Autodesk Inventor part; units mm, degrees
ref_plane "YZ Plane" through (0, 0, 0) normal (1, 0, 0) x (0, 1, 0)
ref_plane "XZ Plane" through (0, 0, 0) normal (0, 1, 0) x (-1, 0, 0)
ref_plane "XY Plane" through (0, 0, 0) normal (0, 0, 1) x (1, 0, 0)
sketch "Esboço1" plane through (0, 0, 0) normal (0, 0, 1) x (1, 0, 0)
  line L0 (-15, 15) -> (15, 15) construction
  line L1 (-15, 15) -> (-15, 10.6) construction
  line L2 (-15, 10.6) -> (-13, 10.6) construction
  line L3 (-13, 13.6) -> (-13, 10.6) construction
  line L4 (-13, 13.6) -> (-9.4247, 10.6) construction
  line L5 (-9.4247, 10.6) -> (-9.4247, 4.4) construction
  line L6 (-9.4247, 4.4) -> (-13, 1.4) construction
  line L7 (-13, 4.4) -> (-13, 1.4) construction
  line L8 (-15, 4.4) -> (-13, 4.4) construction
  line L9 (-15, 4.4) -> (-15, 0) construction
  line L10 (-15, 0) -> (0, 0) construction
  line L11 (-15, 4.4) -> (-14.5, 4.4) construction
  line L12 (-14.5, 4.4) -> (-14.5, 3.9)
  line L13 (-14.5, 3.9) -> (-15, 3.9)
  line L14 (-15, 3.9) -> (-15, 4.4) construction
  line L15 (-15, 10.6) -> (-14.5, 10.6) construction
  line L16 (-14.5, 10.6) -> (-14.5, 11.1)
  line L17 (-14.5, 11.1) -> (-15, 11.1)
  line L18 (-15, 11.1) -> (-15, 10.6) construction
  line L19 (-3.1, 9.4247) -> (3.1, 9.4247) construction
  line L20 (-6.1, 13) -> (-3.1, 9.4247) construction
  line L21 (-6.1, 13) -> (-3.1, 13) construction
  line L22 (-3.1, 15) -> (-3.1, 13) construction
  line L23 (-3.1, 9.4247) -> (0, 9.4247) construction
  line L24 (-3.1, 15) -> (-3.6, 15) construction
  line L25 (-3.6, 15) -> (-3.6, 14.5)
  line L26 (-3.6, 14.5) -> (-3.1, 14.5)
  line L27 (-3.1, 14.5) -> (-3.1, 15) construction
  line L28 (-9.4247, 2) -> (0, 2) construction
  line L29 (-7.4247, 3.6782) -> (-9.4247, 2) construction
  line L30 (-7.4247, 10.6) -> (-7.4247, 3.6782) construction
  line L31 (-7.4247, 10.6) -> (-4.944, 7.4247) construction
  line L32 (-4.944, 7.4247) -> (0, 7.4247) construction
  arc A0 (-14.5, 15) -> (-15, 14.5) centre (-14.5, 14.5) ccw
  arc A1 (-12.1786, 12.9108) -> (-13, 12.5277) centre (-12.5, 12.5277) ccw
  line L33 (-13, 12.5277) -> (-13, 10.6)
  line L34 (-13, 10.6) -> (-14.5, 10.6)
  arc A2 (-9.4247, 10.3668) -> (-9.6033, 10.7499) centre (-9.9247, 10.3668) ccw
  arc A3 (-9.6033, 4.2501) -> (-9.4247, 4.6332) centre (-9.9247, 4.6332) ccw
  arc A4 (-13, 2.4723) -> (-12.1786, 2.0892) centre (-12.5, 2.4723) ccw
  line L35 (-9.6033, 4.2501) -> (-12.1786, 2.0892)
  line L36 (-13, 2.4723) -> (-13, 4.4)
  arc A5 (-15, 0.5) -> (-14.5, 0) centre (-14.5, 0.5) ccw
  line L37 (-15, 14.5) -> (-15, 11.1)
  line L38 (-15, 3.9) -> (-15, 0.5)
  arc A6 (-8.4247, 2.8391) -> (-8.1193, 2) centre (-8.1193, 2.4751) ccw
  arc A7 (-6.5307, 9.4557) -> (-7.4247, 9.1479) centre (-6.9247, 9.1479) ccw
  line L39 (-8.1193, 2) -> (0, 2)
  arc A8 (-7.6033, 3.5283) -> (-7.4247, 3.9114) centre (-7.9247, 3.9114) ccw
  arc A9 (-5.0941, 7.6169) -> (-4.7001, 7.4247) centre (-4.7001, 7.9247) ccw
  arc A10 (-3.2499, 9.6033) -> (-2.8668, 9.4247) centre (-2.8668, 9.9247) ccw
  arc A11 (-5.0277, 13) -> (-5.4108, 12.1786) centre (-5.0277, 12.5) ccw
  line L40 (-5.0277, 13) -> (-3.1, 13)
  line L41 (-2.8668, 9.4247) -> (0, 9.4247)
  line L42 (-4.7001, 7.4247) -> (0, 7.4247)
  line L43 (-6.5307, 9.4557) -> (-5.0941, 7.6169)
  line L44 (-7.4247, 9.1479) -> (-7.4247, 3.9114)
  line L45 (0, 2) -> (0, 0)
  line L46 (0, 7.4247) -> (0, 9.4247)
  line L47 (-3.1, 14.5) -> (-3.1, 13)
  line L48 (-14.5, 4.4) -> (-13, 4.4)
  line L49 (-8.4247, 2.8391) -> (-7.6033, 3.5283)
  line L50 (-14.5, 15) -> (-3.6, 15)
  line L51 (-12.1786, 12.9108) -> (-9.6033, 10.7499)
  line L52 (-9.4247, 10.3668) -> (-9.4247, 4.6332)
  line L53 (-14.5, 0) -> (0, 0)
  line L54 (-5.4108, 12.1786) -> (-3.2499, 9.6033)
  point P0 (0, 15)
  point P1 (-14, 4.4)
  point P2 (-1.55, 9.4247)
  point P3 (-7.25, 0)
  dimension "d0" = 30
  dimension "d1" = 15
  dimension "d6" = 2
  dimension "d7" = 3
  dimension "d9" = 50
  dimension "d12" = 0.5
  dimension "d18" = 50
  dimension "d19" = 2
  dimension "d21" = 2
  dimension "d22" = 2
  dimension "d24" = 2
  dimension "d25" = 0.5
  dimension "d26" = 0.5
  dimension "d27" = 0.5
  dimension "d28" = 0.5
  dimension "d29" = 0.5
  dimension "d30" = 0.5
  dimension "d31" = 0.5
  dimension "d32" = 0.5
  dimension "d33" = 0.5
  dimension "d34" = 0.5
  dimension "d35" = 0.5
  dimension "d38" = 3.1
  dimension "d39" = 6.2
  dimension "d40" = 15
extrude "Extrusão1" add sketch "Esboço1" along normal mid plane 50
mirror "Espelhar1" about plane through (0, 0, 0) normal (1, 0, 0) of "Extrusão1"
equation "\"d6\" = d21"
equation "\"d18\" = d9"
equation "\"d19\" = d21"
equation "\"d22\" = d20"
equation "\"d24\" = d21"
equation "\"d25\" = d35"
equation "\"d26\" = d35"
equation "\"d27\" = d35"
equation "\"d28\" = d35"
equation "\"d29\" = d35"
equation "\"d30\" = d35"
equation "\"d31\" = d35"
equation "\"d32\" = d35"
equation "\"d33\" = d35"
equation "\"d34\" = d35"
equation "\"d39\" = 2 * d38"
properties part number "perfil_15x30_001" material "Alumínio 6061"
Geometry check sheet. Reference: the model listing, model coordinates, mm. A direction names the side the tool comes from. Round coordinates to 2 decimals unless told otherwise and drop trailing zeros. Write each loop counter-clockwise with the first axis right and the second up, starting at its lowest first coordinate (ties: lowest second). Pieces come first, ordered by that corner, then holes. Notation, with made-up numbers: (-11, 15.25) -> (39, 15.25) arc R18 ccw to (39, 22.25) -> close; hole circle Ø6 at (-26.5, 64.5). An arc over 180 degrees is marked (long way). One line per item, written item: value. Start each with the question number.
(1) Draft check along X on faces 6 (the flat face through (4.315, 10.873, -0.35)), 7 (the flat face through (0, 8, -25)), 8 (the flat face through (9.425, 7, 0)). Enter one of: +X half, -X half, draft (parallel to the pull), parting line (faces both ways), or undercut.
(2) Cross-section at B-B, the plane x = -2.25. Record the cut outline in (y, z), and give its area (3 significant figures).
(3) Scan lines: line 1 (Y direction, x = -4.5, z = -18.5); line 2 (X direction, y = 5.5, z = 22.5); line 3 (Y direction, x = -1, z = 22.5). Record each from-to range of solid material in increasing order. Write a range as [from, to].
(4) Go/stop test with flat-tipped pins: pin 1 Ø4.5 at (y, z) = (6.5, 10) entering from -X; pin 2 Ø3 at (y, z) = (6.5, 8.5) entering from +X. Record where each tip stops, or that it passes through.
(5) Cross-section at A-A, the plane y = 6.5. Record the cut outline in (x, z), and give its area (3 significant figures).
(6) Access from +Z, -Z, +X, -X, +Y, -Y to the whole of each face (thin tool, end or side, straight path). Record for faces 1 (the flat face through (15, 13, 0)), 2 (the flat face through (0, 9.425, 0)), 3 (the flat face through (-5.822, 8.549, -0.35)), 4 (the flat face through (14, 10.6, 0)), 5 (the flat face through (-9.425, 8, 0)).
Answer:
1. face 6: undercut
1. face 7: draft
1. face 8: +X half
2. outline: (0, -25) -> (2, -25) -> (2, 25) -> (0, 25) -> close; (7.42, -25) -> (9.42, -25) -> (9.42, 25) -> (7.42, 25) -> close
2. area: 200 mm²
3. line 1: [0, 2], [7.42, 11.09], [13, 15]
3. line 2: [-9.42, -7.42], [7.42, 9.42]
3. line 3: [0, 2], [7.42, 9.42]
4. pin 1: x = -14.5
4. pin 2: x = 9.42
5. outline: (-9.42, -25) -> (-7.42, -25) -> (-7.42, 25) -> (-9.42, 25) -> close; (7.42, -25) -> (9.42, -25) -> (9.42, 25) -> (7.42, 25) -> close
5. area: 200 mm²
6. face 1: +Z, -Z, +X, +Y, -Y
6. face 2: +Z, -Z, +Y
6. face 3: +Z, -Z
6. face 4: +Z, -Z, +X
6. face 5: +Z, -Z, -X
